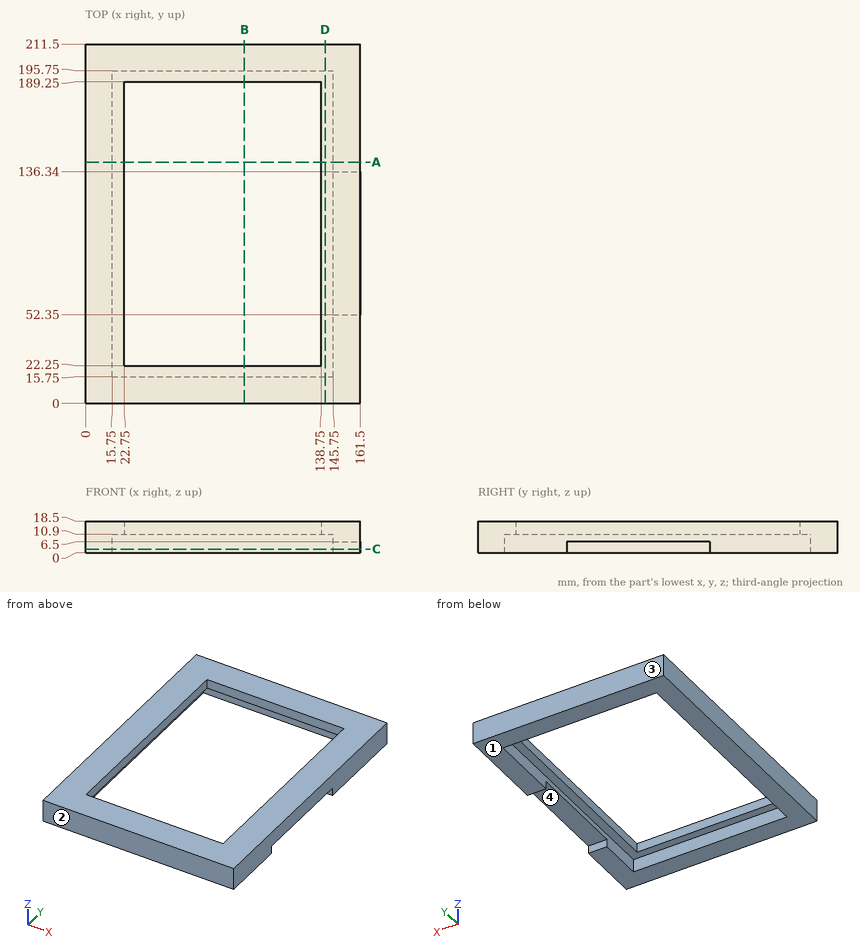
Can you work these out from the drawing? Everything is in mm from the part's minimum corner. Round coordinates to 2 decimals unless told otherwise and drop trailing zeros. Loops run counter-clockwise (first coordinate to the right, second up) from the corner with the lowest first, then second, coordinate; pieces in that order, holes last. Notation, with made-up numbers: (64.25, 12.25) - (113.25, 12.25) arc R16 ccw to (113.25, 18.25) - close; hole circle Ø5 at (-33, -30.75). An arc over 180 degrees is marked (long way). Answer in a Markdown table with one row per item. Add a question column.
(1) I need wall thicknesses on line 1 along X through (y, z) = (128.5, 10.5); line 2 along Y through (x, z) = (115, 16.5); line 3 along Y through (x, z) = (145.5, 10). Which ranges of each line are inside material? Lowest first, please.
(2) If we section it at D-D (x = 141): Please give me the cut outline in (y, z), plus the area to 3 significant figures.
(3) If we section it at C-C (z = 2.25): Please give me the cut outline in (x, y), plus the area to 3 significant figures.
(4) If we mould it in two halves opening along Y, with no side actions, what happens to the marked faces 1, 2, 3 and 4? For each: pulls with the +Y half, pulls with the -Y half, needs draft (parallel to the pull), parting line crosses it, or undercut.
(5) I'm going to push flat-ended pins straight in: pin 1 (3.5 mm diameter, centred on y = 92, z = 3.5, fed in from +X); pin 2 (8 mm diameter, centred on x = 154.5, y = 79, fed in from -Z). Where does each tip first touch, or does it pass through?
(6) If we section it at B-B (x = 93.5): Please give me the cut outline in (y, z).
(7) If we section it at A-A (y = 142): Please give me the cut outline in (x, z).
Model answer:
| question | item | result |
|---|---|---|
| 1 | line 1 | x = 0 to 15.75, 145.75 to 161.5 |
| 1 | line 2 | y = 0 to 22.25, 189.25 to 211.5 |
| 1 | line 3 | y = 0 to 15.75, 195.75 to 211.5 |
| 2 | outline | (0, 0) - (15.75, 0) - (15.75, 10.9) - (195.75, 10.9) - (195.75, 0) - (211.5, 0) - (211.5, 18.5) - (0, 18.5) - close |
| 2 | area | 1,950 mm² |
| 3 | outline | (0, 0) - (161.5, 0) - (161.5, 52.35) - (145.75, 52.35) - (145.75, 15.75) - (15.75, 15.75) - (15.75, 195.75) - (145.75, 195.75) - (145.75, 136.34) - (161.5, 136.34) - (161.5, 211.5) - (0, 211.5) - close |
| 3 | area | 9,430 mm² |
| 4 | face 1 | needs draft |
| 4 | face 2 | pulls with the -Y half |
| 4 | face 3 | pulls with the +Y half |
| 4 | face 4 | undercut |
| 5 | pin 1 | stops at x = 15.75 |
| 5 | pin 2 | stops at z = 6.5 |
| 6 | outline | (0, 0) - (15.75, 0) - (15.75, 10.9) - (22.25, 10.9) - (22.25, 18.5) - (0, 18.5) - close; (189.25, 10.9) - (195.75, 10.9) - (195.75, 0) - (211.5, 0) - (211.5, 18.5) - (189.25, 18.5) - close |
| 7 | outline | (0, 0) - (15.75, 0) - (15.75, 10.9) - (22.75, 10.9) - (22.75, 18.5) - (0, 18.5) - close; (138.75, 10.9) - (145.75, 10.9) - (145.75, 0) - (161.5, 0) - (161.5, 18.5) - (138.75, 18.5) - close |
